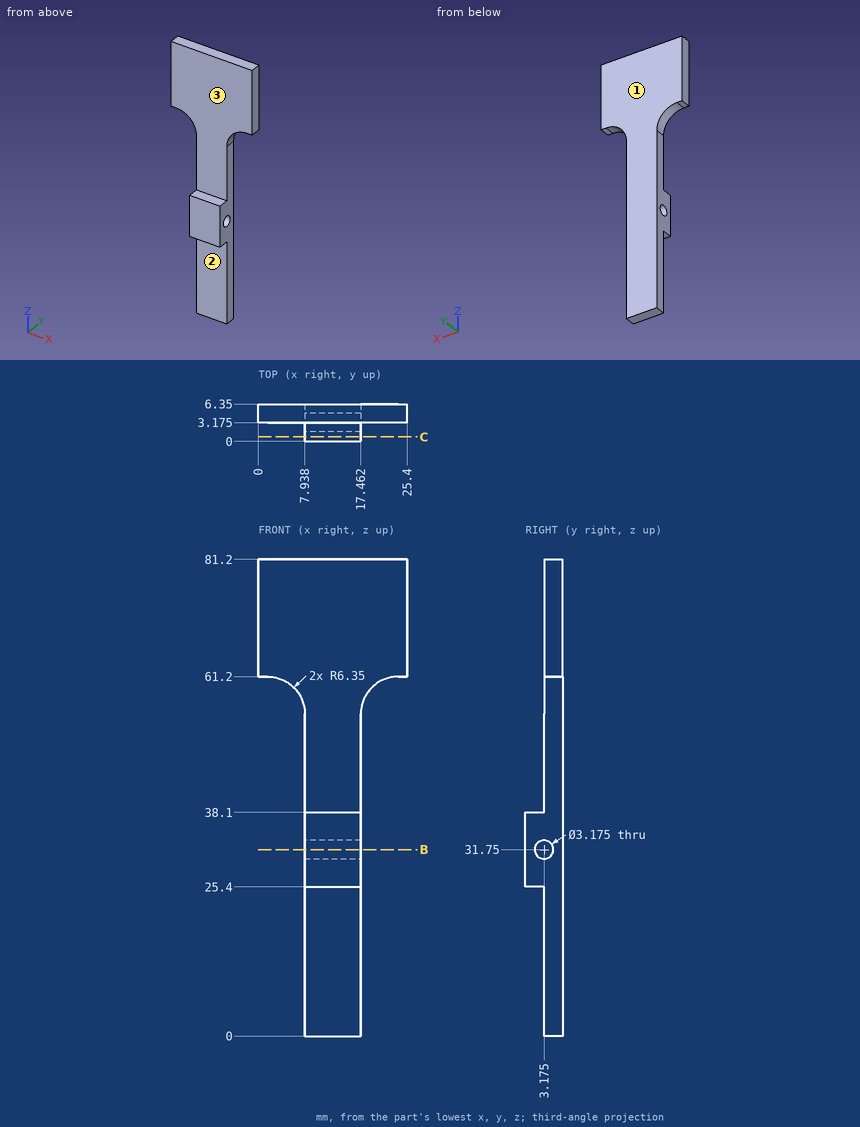
Drawing for the job (mm, zero at the part's lowest x, y, z). A direction names the side the tool comes from. Round coordinates to 2 decimals unless told otherwise and drop trailing zeros. Loops run counter-clockwise (first coordinate to the right, second up) from the corner with the lowest first, then second, coordinate; pieces in that order, holes last. Notation, with made-up numbers: (-23.75, 60.25) -> (-0.75, 60.25) arc R35 ccw to (-0.75, 96.25) -> close; hole circle Ø3 at (45, -25.75). An arc over 180 degrees is marked (long way). Answer as CSV lines item,"result". Start each with the question number.
1) Slice it at C-C (y = 0.75). List the corners of the cut face in (x, z), plus the area to 3 significant figures.
2) Tool access for the marked faces 1, 2 and 3: list every direction of +Z, -Z, +X, -X, +Y, -Y with a clear straight run to the whole face (end or side of a thin tool).
3) Pin check, flat tips, straight feed: P1, Ø1, axis at x = 14, y = 2, coming from the -Z side; P2, Ø2.5, axis at x = 12, y = 1, coming from the +Z side; P3, Ø1.7, axis at x = 24.5, y = 4, coming from the -Z side. Stop position of each tip, or through.
4) Probe line 1 along Y through (x, z) = (10.75, 31.75); line 2 along Z through (x, y) = (10.25, 0.75); line 3 along X through (y, z) = (4, 28.5). List the from-to ranges inside material, lowest first.
5) Slice it at B-B (z = 31.75). List the corners of the cut face in (x, y).
Filled in:
1,outline,"(7.94, 25.4) -> (17.46, 25.4) -> (17.46, 38.1) -> (7.94, 38.1) -> close"
1,area,"121 mm2"
2,face 1,"+Z, -Z, +X, -X, +Y"
2,face 2,"-Z, +X, -X, -Y"
2,face 3,"+Z, +X, -X, -Y"
3,P1,"stops at z = 25.4"
3,P2,"stops at z = 38.1"
3,P3,"stops at z = 61.2"
4,line 1,"y = 0 to 1.59, 4.76 to 6.35"
4,line 2,"z = 25.4 to 38.1"
4,line 3,"x = 7.94 to 17.46"
5,outline,"(7.94, 0) -> (17.46, 0) -> (17.46, 1.59) -> (7.94, 1.59) -> close; (7.94, 4.76) -> (17.46, 4.76) -> (17.46, 6.35) -> (7.94, 6.35) -> close"
